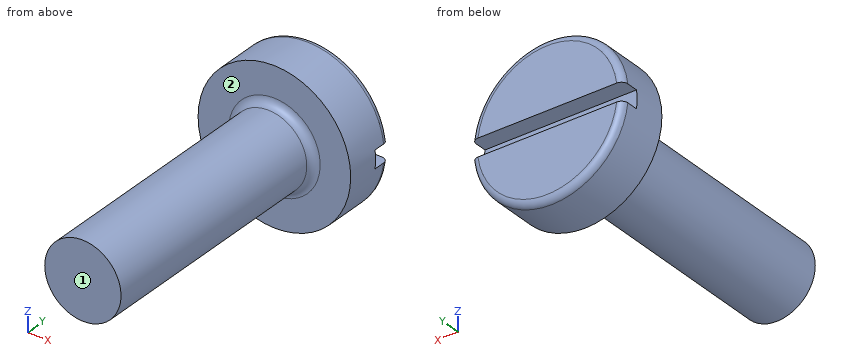
Autodesk Inventor part; units mm, degrees
ref_plane "YZ Plane" through (0, 0, 0) normal (1, 0, 0) x (0, 1, 0)
ref_plane "XZ Plane" through (0, 0, 0) normal (0, 1, 0) x (-1, 0, 0)
ref_plane "XY Plane" through (0, 0, 0) normal (0, 0, 1) x (1, 0, 0)
sketch "Sketch1" plane through (0, 0, 0) normal (0, 0, 1) x (1, 0, 0)
  line L0 (0, 0) -> (-1.5, 0)
  line L1 (-1.5, 0) -> (-1.5, 9)
  line L2 (-1.5, 9) -> (-1.5, 9)
  line L3 (-1.5, 9) -> (-1.5, 10)
  line L4 (-1.5, 10) -> (-3, 10)
  line L5 (-3, 10) -> (-3, 12)
  line L6 (-3, 12) -> (0, 12)
  line L7 (0, 12) -> (0, 0)
  dimension "d0" = 2
  dimension "d1" = 3
  dimension "d2" = 1.5
  dimension "d3" = 0
  dimension "d4" = 1
  dimension "d5" = 12
  dimension "d6" = 90
revolve "Revolution1" add sketch "Sketch1" angle 360 about axis through (0, 12, 0) along (0, -1, 0)
thread "Thread1"
sketch "Sketch2" plane through (0, 12, 0) normal (0, 1, 0) x (1, 0, 0)
  line L0 (5, 0.35) -> (-5, 0.35)
  line L1 (-5, 0.35) -> (-5, -0.35)
  line L2 (-5, -0.35) -> (5, -0.35)
  line L3 (5, -0.35) -> (5, 0.35)
  line L4 (5, 0.35) -> (-5, -0.35) construction
  line L5 (-5, 0.35) -> (5, -0.35) construction
  point P0 (0, 0)
  dimension "d10" = 10
  dimension "d11" = 0.7
fillet "Fillet1" radius 0.25 1 edges at (3, 12, 0)
extrude "Extrusion2" cut sketch "Sketch2" against normal blind 0.7
fillet "Fillet2" radius 0.3 1 edges at (1.5, 10, 0)
properties part number "Screw-CheeseHead-Brass-M3x10-Fine" material "Brass, Soft Yellow"
The listing builds one solid part. Answer for the finished solid, in the listing's coordinates (mm). Face numbers are marked on the shaded views. A direction names the side the tool comes from. Coordinates: 2 decimals unless noted, no trailing zeros. Order: outer loops, then holes, each group sorted by start corner. A loop starts at its lowest first (then second) coordinate and runs counter-clockwise, first axis right, second up.
Q1. Consider line 1 (Y direction, x = 0.5, z = -2.25); line 2 (Z direction, x = -0.1, y = 10.75); line 3 (Z direction, x = 0.05, y = 4.25). Determine where each line is inside the solid, lowest interval first.
Q2. Which of the six approach directions +Z, -Z, +X, -X, +Y, -Y give full straight-line access (tool end or side, diameter ignored) to the marked faces 1 and 2?
Q3. A cutting plane is placed at B-B, the plane z = 0. Write down the section's boundary in (x, y).
Q4. A cutting plane is placed at D-D, the plane y = 10.75. Write down the section's boundary in (x, z), and give its area (3 significant figures).
Q5. A cutting plane is placed at C-C, the plane y = 1.5. Write down the section's boundary in (x, z).
Q6. A cutting plane is placed at A-A, the plane x = 0. Write down the section's boundary in (y, z).
Q7. Given P1, Ø0.6, axis at x = 0.5, z = 0, coming from the +Y side, flat-ended and moving along its own axis, determine where the tip first touches the part or whether it passes through.
Answers follow:
1. line 1: y = 10 to 12
1. line 2: z = -3 to 3
1. line 3: z = -1.5 to 1.5
2. face 1: +Z, -Z, +X, -X, -Y
2. face 2: -Y
3. outline: (-3, 10) - (-1.8, 10) arc R0.3 cw to (-1.5, 9.7) - (-1.5, 0) - (1.5, 0) - (1.5, 9.7) arc R0.3 cw to (1.8, 10) - (3, 10) - (3, 11.3) - (-3, 11.3) - close
4. outline: circle Ø6 at (0, 0)
4. area: 28.3 mm2
5. outline: circle Ø3 at (0, 0)
6. outline: (0, -1.5) - (9.7, -1.5) arc R0.3 cw to (10, -1.8) - (10, -3) - (11.75, -3) arc R0.25 ccw to (12, -2.75) - (12, -0.35) - (11.3, -0.35) - (11.3, 0.35) - (12, 0.35) - (12, 2.75) arc R0.25 ccw to (11.75, 3) - (10, 3) - (10, 1.8) arc R0.3 cw to (9.7, 1.5) - (0, 1.5) - close
7. P1: stops at y = 11.3
